Could you check a few things on this model? Use its own coordinates, in mm. Face numbers are marked on the shaded views. A direction names the side the tool comes from. Round coordinates to 2 decimals unless told otherwise and drop trailing zeros. Order: outer loops, then holes, each group sorted by start corner. A loop starts at its lowest first (then second) coordinate and runs counter-clockwise, first axis right, second up. Notation, with made-up numbers: (27.5, 16) - (66.5, 16) arc R16 ccw to (66.5, 21) - close; hole circle Ø5 at (76, 9.5). An arc over 180 degrees is marked (long way). Use one line per item in the form item = value.
from build123d import *

# Parameters (mm, degrees)
SKETCH1_R           = 30
BOSS_EXTRUDE1_DEPTH = 22


with BuildPart() as part:
    # Sketch1 → Boss-Extrude1 (new body)
    with BuildSketch(Plane(origin=(0, 0, 0), x_dir=(0, 0, -1), z_dir=(1, 0, 0))):
        Circle(SKETCH1_R)
        Polygon((-16.541112452, 22.766888123), (-10.26013758, 21.772079433), (-4.496681536, 23.64473982), (0, 28.141421356), (4.496681536, 23.64473982), (10.26013758, 21.772079433), (16.541112452, 22.766888123), (17.535921141, 16.485913251), (21.09793287, 11.583224708), (26.764082159, 8.696177445), (23.877034895, 3.030028156), (23.877034895, -3.030028156), (26.764082159, -8.696177445), (21.09793287, -11.583224708), (17.535921141, -16.485913251), (16.541112452, -22.766888123), (10.26013758, -21.772079433), (4.496681536, -23.64473982), (0, -28.141421356), (-4.496681536, -23.64473982), (-10.26013758, -21.772079433), (-16.541112452, -22.766888123), (-17.535921141, -16.485913251), (-21.09793287, -11.583224708), (-26.764082159, -8.696177445), (-23.877034895, -3.030028156), (-23.877034895, 3.030028156), (-26.764082159, 8.696177445), (-21.09793287, 11.583224708), (-17.535921141, 16.485913251), align=None, mode=Mode.SUBTRACT)
    extrude(amount=BOSS_EXTRUDE1_DEPTH)


solid = part.part
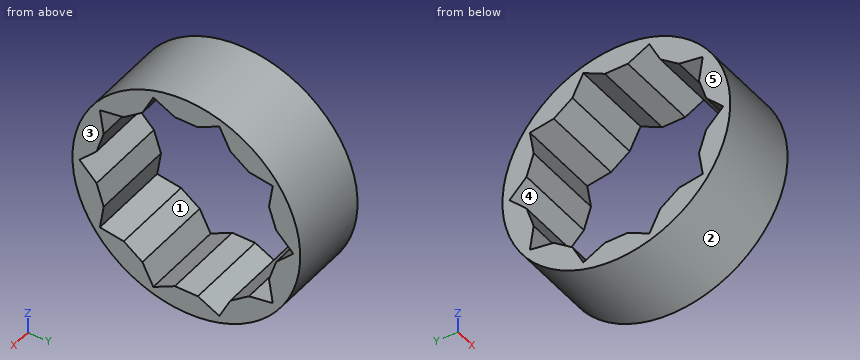
Item 1: I need wall thicknesses on L1, parallel to Y at x = 5, z = 24; L2, parallel to Y at x = 4.75, z = -26; L3, parallel to Y at x = 15.75, z = 16. Which ranges of each line are inside material? Lowest first, please.
Found:
L1 = -18 to -10.1, -3.27 to 3.27, 10.1 to 18
L2 = -14.97 to -9.09, -7.2 to 7.2, 9.09 to 14.97
L3 = -25.38 to -22.68, 22.68 to 25.38
Item 2: Will these pins go through, and if not, where does the flat tip stop? P1, Ø3, axis at x = 5.5, z = -6.5, coming from the -Y side; P2, Ø6, axis at x = 16.5, z = -17, coming from the -Y side; P3, Ø1, axis at x = 2.5, y = -18.5, coming from the -Z side.
Found:
P1 = -29.58
P2 = -26.53
P3 = -24
Item 3: Imagine slicing it at C-C on y = -19.5. Please give me the cut outline in (x, z).
Found:
outline = (0, -22.8) - (22, -22.8) - (22, -17.06) - (0, -17.06) - close; (0, 17.06) - (22, 17.06) - (22, 22.8) - (0, 22.8) - close
Item 4: If we mould it in two halves opening along Y, with no side actions, what happens to the marked faces 1, 2 and 3? For each: released by +Y, released by -Y, zero draft, split by the parting line, or undercut.
Found:
face_1 = undercut
face_2 = split by the parting line
face_3 = zero draft
Item 5: Imagine slicing it at A-A on y = 0. Please give me the cut outline in (x, z).
Found:
outline = (0, -30) - (22, -30) - (22, -23.88) - (0, -23.88) - close; (0, 23.88) - (22, 23.88) - (22, 30) - (0, 30) - close
Item 6: For the marked faces 4 and 5, which set-ups out of +Z, -Z, +X, -X, +Y, -Y let a thin tool reach every point of the face, with its end or its side?
Found:
face_4 = +X, -X
face_5 = +Z, -Z, -X, +Y, -Y
